from build123d import *

# Parameters (mm, degrees)
F1_DEPTH = 3


with BuildPart() as f1:
    # F0 (on Front) → F1 (new body)
    with BuildSketch(Plane.XZ):
        Polygon((167.500045, -126.000002), (167.500045, 123.999998), (150.500045, 123.999998), (150.500045, 120.999998), (133.500045, 120.999998), (133.500045, 123.999998), (116.500045, 123.999998), (116.500045, 120.999998), (99.500045, 120.999998), (99.500045, 123.999998), (82.500045, 123.999998), (82.500045, 120.999998), (65.500045, 120.999998), (65.500045, 123.999998), (48.500045, 123.999998), (48.500045, 120.999998), (31.500045, 120.999998), (31.500045, 123.999998), (14.500045, 123.999998), (14.500045, 120.999998), (-2.499955, 120.999998), (-2.499955, 123.999998), (-19.499955, 123.999998), (-19.499955, 120.999998), (-36.499955, 120.999998), (-36.499955, 123.999998), (-53.499955, 123.999998), (-53.499955, 120.999998), (-70.499955, 120.999998), (-70.499955, 123.999998), (-87.499955, 123.999998), (-87.499955, 120.999998), (-104.499955, 120.999998), (-104.499955, 123.999998), (-121.499955, 123.999998), (-121.499955, 120.999998), (-138.499955, 120.999998), (-138.499955, 123.999998), (-155.499955, 123.999998), (-155.499955, 120.999998), (-169.499955, 120.999998), (-169.499955, 108.374998), (-172.499955, 108.374998), (-172.499955, 92.749998), (-169.499955, 92.749998), (-169.499955, 77.124998), (-172.499955, 77.124998), (-172.499955, 61.499998), (-169.499955, 61.499998), (-169.499955, 45.874998), (-172.499955, 45.874998), (-172.499955, 30.249998), (-169.499955, 30.249998), (-169.499955, 14.624998), (-172.499955, 14.624998), (-172.499955, -1.000002), (-169.499955, -1.000002), (-169.499955, -16.625002), (-172.499955, -16.625002), (-172.499955, -32.250002), (-169.499955, -32.250002), (-169.499955, -47.875002), (-172.499955, -47.875002), (-172.499955, -63.500002), (-169.499955, -63.500002), (-169.499955, -79.125002), (-172.499955, -79.125002), (-172.499955, -94.750002), (-169.499955, -94.750002), (-169.499955, -110.375002), (-172.499955, -110.375002), (-172.499955, -123.000002), (-155.499955, -123.000002), (-155.499955, -126.000002), (-138.499955, -126.000002), (-138.499955, -123.000002), (-121.499955, -123.000002), (-121.499955, -126.000002), (-104.499955, -126.000002), (-104.499955, -123.000002), (-87.499955, -123.000002), (-87.499955, -126.000002), (-70.499955, -126.000002), (-70.499955, -123.000002), (-53.499955, -123.000002), (-53.499955, -126.000002), (-36.499955, -126.000002), (-36.499955, -123.000002), (-19.499955, -123.000002), (-19.499955, -126.000002), (-2.499955, -126.000002), (-2.499955, -123.000002), (14.500045, -123.000002), (14.500045, -126.000002), (31.500045, -126.000002), (31.500045, -123.000002), (48.500045, -123.000002), (48.500045, -126.000002), (65.500045, -126.000002), (65.500045, -123.000002), (82.500045, -123.000002), (82.500045, -126.000002), (99.500045, -126.000002), (99.500045, -123.000002), (116.500045, -123.000002), (116.500045, -126.000002), (133.500045, -126.000002), (133.500045, -123.000002), (150.500045, -123.000002), (150.500045, -126.000002), align=None)
    extrude(amount=F1_DEPTH)


solid = f1.part
For this review, take the finished solid that the model builds, in its own axes (mm). Coordinates: 2 decimals unless noted, no trailing zeros. Loops run counter-clockwise (first coordinate to the right, second up) from the corner with the lowest first, then second, coordinate; pieces in that order, holes last. Notation, with made-up numbers: (-11.5, 38) - (-7.5, 38) arc R11 ccw to (-7.5, 59) - close; hole circle Ø10 at (-33.5, 75). An arc over 180 degrees is marked (long way). Return JSON: item names as keys, results as strings.
Item 1: Take a section at A-A (x = 111). Give the boundary of the cut face in (y, z).
Determined:
{"outline": "(-3, -123) - (0, -123) - (0, 121) - (-3, 121) - close"}
Item 2: Insertion check: pin 1 (1.5 mm diameter, centred on y = -1.5, z = -125, fed in from -X); pin 2 (0.9 mm diameter, centred on x = -171, y = -1, fed in from -Z); pin 3 (0.9 mm diameter, centred on x = -26, y = -2, fed in from +Z). Each pin has a flat end and moves straight along its axis. Give the tip position at first contact, or say it passes through.
Determined:
{"pin 1": "stops at x = -155.5", "pin 2": "stops at z = -123", "pin 3": "stops at z = 121"}
Item 3: For line 1 (Z direction, x = -133.5, y = -1.25); line 2 (X direction, y = -1.3, z = -109), list the stretches that pass through material, from the lowest coordinate up.
Determined:
{"line 1": "z = -123 to 121", "line 2": "x = -169.5 to 167.5"}
